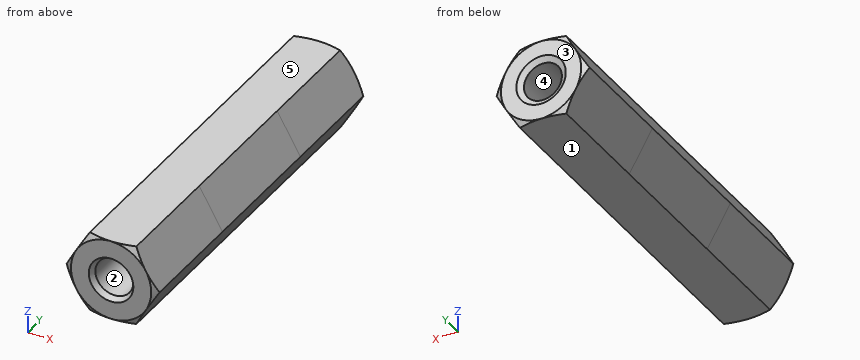
```python
from build123d import *

# Parameters (mm, degrees)
SKETCH1_R             = 4.041451884
SKETCH1_R_2           = 1.65
BOSS_EXTRUDE1_DEPTH   = 32
CHAMFER1_SIZE         = 0.55
CHAMFER1_SIZE2        = 0.317542648
CHAMFER2_SIZE         = 0.55
CHAMFER2_SIZE2        = 0.317542648
SKETCH2_OUTSIDE_W     = 16.878
SKETCH2_OUTSIDE_H     = 16.878
CUT_EXTRUDE1_DEPTH    = 33
CHAMFER3_SIZE         = 0.5
CHAMFER3_SIZE2        = 0.288675135
CHAMFER3_PART_2_SIZE  = 0.5
CHAMFER3_PART_2_SIZE2 = 0.288675135
SKETCH3_W             = 4.041451884
SKETCH3_H             = 12
BOSS_EXTRUDE2_DEPTH   = 7


with BuildPart() as part:
    # Sketch1 → Boss-Extrude1 (new body)
    with BuildSketch(Plane(origin=(0, 0, 0), x_dir=(1, 0, 0), z_dir=(0, 1, 0))):
        Circle(SKETCH1_R)
        Circle(SKETCH1_R_2, mode=Mode.SUBTRACT)
    extrude(amount=BOSS_EXTRUDE1_DEPTH)

    # Chamfer1
    chamfer1_edges = [part.edges().sort_by_distance(p)[0] for p in [
        (-4.041451884, 32, 0),
    ]]
    chamfer1_side = [part.faces().sort_by_distance(p)[0] for p in [
        (-3.927142363, 32, 0),
    ]]
    chamfer(chamfer1_edges, length=CHAMFER1_SIZE, length2=CHAMFER1_SIZE2, reference=chamfer1_side[0])

    # Chamfer2
    chamfer2_edges = [part.edges().sort_by_distance(p)[0] for p in [
        (-4.041451884, 0, 0),
    ]]
    chamfer2_side = [part.faces().sort_by_distance(p)[0] for p in [
        (-3.927142363, 0, 0),
    ]]
    chamfer(chamfer2_edges, length=CHAMFER2_SIZE, length2=CHAMFER2_SIZE2, reference=chamfer2_side[0])

    # Sketch2 outside → Cut-Extrude1 (cut, through all)
    with BuildSketch(Plane.XZ):
        Rectangle(SKETCH2_OUTSIDE_W, SKETCH2_OUTSIDE_H)
        Polygon((4.041451884, 0), (2.020725942, -3.5), (-2.020725942, -3.5), (-4.041451884, 0), (-2.020725942, 3.5), (2.020725942, 3.5), align=None, mode=Mode.SUBTRACT)
    extrude(amount=-CUT_EXTRUDE1_DEPTH, mode=Mode.SUBTRACT)

    # Chamfer3
    chamfer3_edges = [part.edges().sort_by_distance(p)[0] for p in [
        (-1.65, 0, 0),
    ]]
    chamfer3_side = [part.faces().sort_by_distance(p)[0] for p in [
        (-1.65, 16, 0),
    ]]
    chamfer(chamfer3_edges, length=CHAMFER3_SIZE, length2=CHAMFER3_SIZE2, reference=chamfer3_side[0])

    # Chamfer3 part 2
    chamfer3_part_2_edges = [part.edges().sort_by_distance(p)[0] for p in [
        (-1.65, 32, 0),
    ]]
    chamfer3_part_2_side = [part.faces().sort_by_distance(p)[0] for p in [
        (-3.392698712, 32, 0),
    ]]
    chamfer(chamfer3_part_2_edges, length=CHAMFER3_PART_2_SIZE, length2=CHAMFER3_PART_2_SIZE2, reference=chamfer3_part_2_side[0])

    # Sketch3 → Boss-Extrude2 (add)
    with BuildSketch(Plane(origin=(-3.031088913, 0, -1.75), x_dir=(-0.5, 0, 0.866025404), z_dir=(-0.866025404, 0, -0.5))):
        with Locations((0, 16)):
            Rectangle(SKETCH3_W, SKETCH3_H)
    extrude(amount=-BOSS_EXTRUDE2_DEPTH)


solid = part.part
```
The listing builds one solid part. Answer for the finished solid, in the listing's coordinates (mm). Face numbers are marked on the shaded views. A direction names the side the tool comes from. Give positions to 0.01 mm unless a question says otherwise; leave off trailing zeros. Order: outer loops, then holes, each group sorted by start corner. A loop starts at its lowest first (then second) coordinate and runs counter-clockwise, first axis right, second up. Notation, with made-up numbers: (2, 18.25) -> (59, 18.25) arc R27 ccw to (59, 50.25) -> close; hole circle Ø3 at (2, 15). An arc over 180 degrees is marked (long way). One line per item, written item: value.
1) A tool of negligible diameter and unlimited length cuts with its end or side. For the marked faces 4 and 5, from which of +Z, -Z, +X, -X, +Y, -Y can it reach the whole face along a straight path? Write none if from no direction.
Reported:
face 4: +Y
face 5: +Z, +X, -X, +Y, -Y
2) Find section C-C, the plane y = 18. Determine the outline of the cut face in (x, z).
Reported:
outline: (-4.04, 0) -> (-2.02, -3.5) -> (2.02, -3.5) -> (4.04, 0) -> (2.02, 3.5) -> (-2.02, 3.5) -> close
3) Find the intervals of material crossed by line 1 (Z direction, x = 0, y = 26.5); line 2 (Y direction, x = 0, z = -0.75); line 3 (X direction, y = 25.5, z = 1), in increasing order.
Reported:
line 1: z = -3.5 to -1.65, 1.65 to 3.5
line 2: y = 10 to 22
line 3: x = -3.46 to -1.31, 1.31 to 3.46
4) Find section A-A, the plane y = 8. Determine the outline of the cut face in (x, z).
Reported:
outline: (-4.04, 0) -> (-2.02, -3.5) -> (2.02, -3.5) -> (4.04, 0) -> (2.02, 3.5) -> (-2.02, 3.5) -> close; hole circle Ø3.3 at (0, 0)
5) Flat-ended cylindrical pins translate along their axes: P1, Ø2, axis at x = 0, z = 0, coming from the -Y side; P2, Ø1.6, axis at x = -0.5, z = 0, coming from the +Y side. Find the tip coordinate at first contact, or state that the pin passes through.
Reported:
P1: stops at y = 10
P2: stops at y = 22
6) Determine the mould class of the marked faces 1, 2 and 3 for opening direction Z: pulls with the +Z half, pulls with the -Z half, needs draft (parallel to the pull), parting line crosses it, or undercut.
Reported:
face 1: pulls with the -Z half
face 2: undercut
face 3: needs draft
